Source: CAD feature listing. Evaluate the final solid. Frame: model axes, mm. Coordinates: 2 decimals unless noted, no trailing zeros. Order: outer loops, then holes, each group sorted by start corner. A loop starts at its lowest first (then second) coordinate and runs counter-clockwise, first axis right, second up.
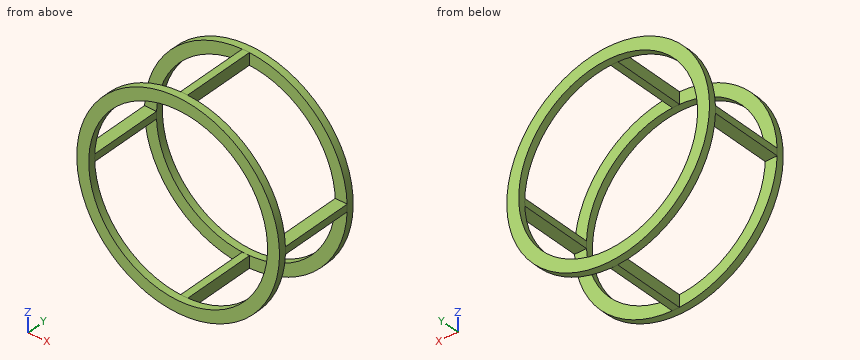
```python
from build123d import *

# Parameters (mm, degrees)
SKETCH1_R           = 53.975
SKETCH1_R_2         = 47.625
BOSS_EXTRUDE1_DEPTH = 3.81
SKETCH2_R           = 53.975
SKETCH2_R_2         = 47.625
BOSS_EXTRUDE2_DEPTH = 3.81
SKETCH4_W           = 6.35
SKETCH4_H           = 39.15918
BOSS_EXTRUDE3_DEPTH = 1.905
CIRPATTERN1_COUNT   = 4


with BuildPart() as part:
    # Sketch1 → Boss-Extrude1 (new body)
    with BuildSketch(Plane(origin=(0, 0, 0), x_dir=(1, 0, 0), z_dir=(0, 1, 0))):
        with Locations(Location((0, 0, 0), (0, 0, 90))):
            Circle(SKETCH1_R)
        with Locations(Location((0, 0, 0), (0, 0, 90))):
            Circle(SKETCH1_R_2, mode=Mode.SUBTRACT)
    extrude(amount=BOSS_EXTRUDE1_DEPTH)



with BuildPart() as body_2:
    # Sketch2 → Boss-Extrude2 (new body)
    with BuildSketch(Plane(origin=(0, 42.96918, 0), x_dir=(1, 0, 0), z_dir=(0, 1, 0))):
        with Locations(Location((0, 0, 0), (0, 0, 90))):
            Circle(SKETCH2_R)
        with Locations(Location((0, 0, 0), (0, 0, 90))):
            Circle(SKETCH2_R_2, mode=Mode.SUBTRACT)
    extrude(amount=BOSS_EXTRUDE2_DEPTH)


with BuildPart() as part_1:
    add(part.part)

    add(body_2.part)  # Boss-Extrude3 merges body 2
    # Sketch4 → Boss-Extrude3 (add, symmetric)
    with BuildSketch(Plane(origin=(0, 0, 0), x_dir=(0, 0, -1), z_dir=(1, 0, 0))):
        with Locations((-50.8, 23.38959)):
            Rectangle(SKETCH4_W, SKETCH4_H)
    boss_extrude3 = extrude(amount=BOSS_EXTRUDE3_DEPTH, both=True)

    # CirPattern1: Boss-Extrude3 ×4 about axis
    cirpattern1_axis = Axis((0, 0, 0), (0, 1, 0))
    for i in range(1, CIRPATTERN1_COUNT):
        add(boss_extrude3.rotate(cirpattern1_axis, i * 360 / CIRPATTERN1_COUNT))


solid = part_1.part
```
1. Pin query (flat end, axial travel): P1, Ø1.9, axis at y = 21, z = -52, coming from the -X side (3 decimals); P2, Ø7, axis at y = 32, z = -49.5, coming from the +X side (3 decimals). Return the tip coordinate at first contact, or that it passes through.
Findings:
P1: stops at x = -1.905
P2: stops at x = 1.905
2. Ray query, line 1 (X direction, y = 45.45, z = 0) (3 decimals); line 2 (Y direction, x = 41.5, z = -30); line 3 (Z direction, x = 36, y = 43). Return the intervals inside material, ascending.
Findings:
line 1: x = -53.975 to -47.625, 47.625 to 53.975
line 2: y = 0 to 3.81, 42.97 to 46.78
line 3: z = -40.22 to -31.18, 31.18 to 40.22
3. Section query B-B on x = 17. Return loops of the section in (y, z), plus the area to 3 significant figures.
Findings:
outline: (0, -51.23) - (3.81, -51.23) - (3.81, -44.49) - (0, -44.49) - close; (0, 44.49) - (3.81, 44.49) - (3.81, 51.23) - (0, 51.23) - close; (42.97, -51.23) - (46.78, -51.23) - (46.78, -44.49) - (42.97, -44.49) - close; (42.97, 44.49) - (46.78, 44.49) - (46.78, 51.23) - (42.97, 51.23) - close
area: 103 mm2
4. Section query A-A on y = 41. Return loops of the section in (x, z) (3 decimals), plus the area to 3 significant figures.
Findings:
outline: (-53.975, -1.905) - (-47.625, -1.905) - (-47.625, 1.905) - (-53.975, 1.905) - close; (-1.905, -53.975) - (1.905, -53.975) - (1.905, -47.625) - (-1.905, -47.625) - close; (-1.905, 47.625) - (1.905, 47.625) - (1.905, 53.975) - (-1.905, 53.975) - close; (47.625, -1.905) - (53.975, -1.905) - (53.975, 1.905) - (47.625, 1.905) - close
area: 96.8 mm2
